from build123d import *

# Parameters (mm, degrees)
ESBO_O1_W                                   = 420
ESBO_O1_H                                   = 70
RESSALTO_EXTRUS_O1_DEPTH                    = 10.7
ESBO_O5_R                                   = 11
CORTE_EXTRUS_O4_DEPTH                       = 7
FURO_ROSCADO_PARA_CONDU_TE_DE_10_321_D      = 5.1054
FURO_ROSCADO_PARA_CONDU_TE_DE_M5X0_81_D     = 5.2
FURO_ROSCADO_PARA_CONDU_TE_DE_1_4_281_D     = 6.6294
FURO_ROSCADO_PARA_CONDU_TE_DE_1_4_281_DEPTH = 15
FURO_ROSCADO_PARA_CONDU_TE_DE_1_4_281_TIP   = 1.991672694


with BuildPart() as part:
    # Esboço1 → Ressalto-extrusão1 (new body)
    with BuildSketch(Plane.XY):
        Rectangle(ESBO_O1_W, ESBO_O1_H)
    extrude(amount=RESSALTO_EXTRUS_O1_DEPTH)

    # Esboço5 → Corte-extrusão4 (cut)
    with BuildSketch(Plane.XY.offset(10.7)):
        with Locations((0, 4.65)):
            Circle(ESBO_O5_R)
    extrude(amount=-CORTE_EXTRUS_O4_DEPTH, mode=Mode.SUBTRACT)

    # Furo roscado para conduíte de #10-321 (through all)
    with Locations(Plane.XY.offset(10.7)):
        with Locations((-170, -5), (-134, -5), (134, -5), (170, -5)):
            Hole(FURO_ROSCADO_PARA_CONDU_TE_DE_10_321_D / 2)

    # Furo roscado para conduíte de M5x0.81 (through all)
    with Locations(Plane.XY.offset(10.7)):
        with Locations((-200, 25), (-200, -25), (200, -25), (200, 25)):
            Hole(FURO_ROSCADO_PARA_CONDU_TE_DE_M5X0_81_D / 2)

    # Furo roscado para conduíte de 1/4-281
    with Locations(Plane(origin=(0, 35, 0), x_dir=(1, 0, 0), z_dir=(0, 1, 0))):
        with Locations((-100, -5.35), (100, -5.35)):
            Hole(FURO_ROSCADO_PARA_CONDU_TE_DE_1_4_281_D / 2, depth=FURO_ROSCADO_PARA_CONDU_TE_DE_1_4_281_DEPTH)
            with Locations((0, 0, -(FURO_ROSCADO_PARA_CONDU_TE_DE_1_4_281_DEPTH + FURO_ROSCADO_PARA_CONDU_TE_DE_1_4_281_TIP / 2))):  # 118° drill point
                Cone(0, FURO_ROSCADO_PARA_CONDU_TE_DE_1_4_281_D / 2, FURO_ROSCADO_PARA_CONDU_TE_DE_1_4_281_TIP, mode=Mode.SUBTRACT)


solid = part.part
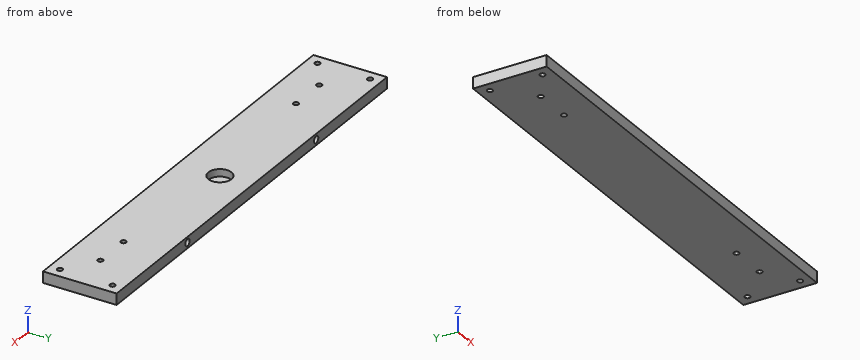
Can you work these out from the model? Positions are in its coordinate system, mm. Coordinates: 2 decimals unless noted, no trailing zeros. Loops run counter-clockwise (first coordinate to the right, second up) from the corner with the lowest first, then second, coordinate; pieces in that order, holes last. Notation, with made-up numbers: M -30.5,11 L 14.5,11 A35 ccw 14.5,50 Z; hole C 44,85 d10. An arc over 180 degrees is marked long. Answer as CSV lines item,"result". Start each with the question number.
1. Suppose I cut it at A-A, the plane y = 4.65. List the corners of the cut face in (x, z) for me.
2. Suppose I cut it at B-B, the plane z = 7. Count the separate pieces of the cut face and the enclosed holes in it, plus the area to 3 significant figures.
3. If I drill on probe 1 along Y at (x, z) = (200, 5); probe 2 along X at (y, z) = (-7, 10); probe 3 along X at (y, z) = (14, 8.25), over which ranges is the centre line in solid material (lowest first)? Write a range as [from, to].
4. For pin 1 Ø3 at (x, y) = (-170, -5) entering from -Z; pin 2 Ø6 at (x, z) = (100, 5.35) entering from +Y, each with a flat end and sliding along its axis, tell me the tip position at first contact or that it passes through.
Output:
1,outline,"M -210,0 L 210,0 L 210,10.7 L 11,10.7 L 11,3.7 L -11,3.7 L -11,10.7 L -210,10.7 Z"
2,separate pieces,"1"
2,enclosed holes,"9"
2,area,"28,700 mm^2"
3,probe 1,"y = [-35, -27.6], [-22.4, 22.4], [27.6, 35]"
3,probe 2,"x = [-210, -171.59], [-168.41, -135.59], [-132.41, 132.41], [135.59, 168.41], [171.59, 210]"
3,probe 3,"x = [-210, -5.79], [5.79, 210]"
4,pin 1,"passes through"
4,pin 2,"stops at y = 19.81"
